Answer from the drawing. Dimensions are ordinates in mm from the lowest x, y and z of the part. A direction names the side the tool comes from. Coordinates: 2 decimals unless noted, no trailing zeros. Write each loop counter-clockwise with the first axis right and the second up, starting at its lowest first coordinate (ties: lowest second). Pieces come first, ordered by that corner, then holes.
1) The part is cut by section D-D (z = 2.25). Determine the outline of the cut face in (x, y).
2) The part is cut by section B-B (x = 54). Determine the outline of the cut face in (y, z), then the cut area to 3 significant figures.
3) The part is cut by section A-A (x = 67.5). Determine the outline of the cut face in (y, z).
4) Determine the mould class of the marked faces 1, 2 and 3 for opening direction X: +X half, -X half, draft (parallel to the pull), parting line (faces both ways), or undercut.
5) The part is cut by section C-C (y = 10). Determine the outline of the cut face in (x, z).
6) Which of the six approach directions +Z, -Z, +X, -X, +Y, -Y give full straight-line access (tool end or side, diameter ignored) to the marked faces 4, 5 and 6?
7) Each of these flat-tipped pins is pushed along its axis until it touches: pin 1 Ø2.5 at (y, z) = (8.5, 3.5) entering from +X; pin 2 Ø4 at (x, y) = (22.5, 10) entering from +Z; pin 3 Ø2.5 at (x, z) = (50.5, 2) entering from +Y; pin 4 Ø2 at (x, y) = (67.5, 10) entering from +Z. Where does it stop, or does it pass through?
8) Find the intervals of material crossed by line 1 (Z direction, x = 59, y = 2.25); line 2 (Y direction, x = 67.5, z = 3.7); line 3 (Y direction, x = 28, z = 13.5), in increasing order.
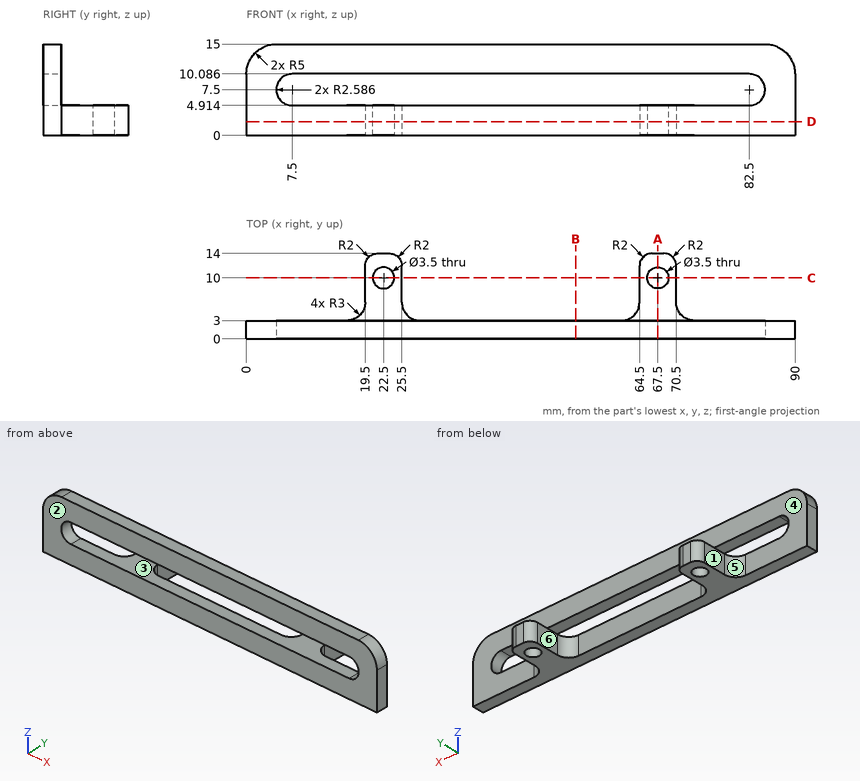
Reported:
1. outline: (0, 0) - (90, 0) - (90, 3) - (73.5, 3) arc R3 cw to (70.5, 6) - (70.5, 12) arc R2 ccw to (68.5, 14) - (66.5, 14) arc R2 ccw to (64.5, 12) - (64.5, 6) arc R3 cw to (61.5, 3) - (28.5, 3) arc R3 cw to (25.5, 6) - (25.5, 12) arc R2 ccw to (23.5, 14) - (21.5, 14) arc R2 ccw to (19.5, 12) - (19.5, 6) arc R3 cw to (16.5, 3) - (0, 3) - close; hole circle Ø3.5 at (22.5, 10); hole circle Ø3.5 at (67.5, 10)
2. outline: (0, 0) - (3, 0) - (3, 4.91) - (0, 4.91) - close; (0, 10.09) - (3, 10.09) - (3, 15) - (0, 15) - close
2. area: 29.5 mm2
3. outline: (0, 0) - (8.25, 0) - (8.25, 4.91) - (0, 4.91) - close; (0, 10.09) - (3, 10.09) - (3, 15) - (0, 15) - close; (11.75, 0) - (14, 0) - (14, 4.91) - (11.75, 4.91) - close
4. face 1: -X half
4. face 2: draft
4. face 3: undercut
5. outline: (19.5, 0) - (20.75, 0) - (20.75, 4.91) - (19.5, 4.91) - close; (24.25, 0) - (25.5, 0) - (25.5, 4.91) - (24.25, 4.91) - close; (64.5, 0) - (65.75, 0) - (65.75, 4.91) - (64.5, 4.91) - close; (69.25, 0) - (70.5, 0) - (70.5, 4.91) - (69.25, 4.91) - close
6. face 4: +Z, +Y
6. face 5: +Z, -Z, -X, +Y
6. face 6: +Z, -Z, +Y
7. pin 1: stops at x = 70.5
7. pin 2: stops at z = 4.91
7. pin 3: stops at y = 3
7. pin 4: passes through
8. line 1: z = 0 to 4.91, 10.09 to 15
8. line 2: y = 0 to 8.25, 11.75 to 14
8. line 3: y = 0 to 3
